Autodesk Inventor part; units mm, degrees
ref_plane "YZ Plane" through (0, 0, 0) normal (1, 0, 0) x (0, 1, 0)
ref_plane "XZ Plane" through (0, 0, 0) normal (0, 1, 0) x (-1, 0, 0)
ref_plane "XY Plane" through (0, 0, 0) normal (0, 0, 1) x (1, 0, 0)
sketch "Sketch1" plane through (0, 0, 0) normal (0, 0, 1) x (1, 0, 0)
  line L0 (-63.88, 42.74) -> (63.88, 42.74)
  line L1 (63.88, 42.74) -> (63.88, -42.74)
  line L2 (63.88, -42.74) -> (-63.88, -42.74)
  line L3 (-63.88, -42.74) -> (-63.88, 42.74)
  line L4 (63.88, 42.74) -> (-63.88, -42.74) construction
  point P0 (0, 0)
  point P1 (0, 0)
  dimension "d0" = 127.76
  dimension "d1" = 85.48
extrude "Extrusion1" add sketch "Sketch1" along normal blind 15
sketch "Sketch2" plane through (0, 0, 0) normal (0, 0, -1) x (-1, 0, 0)
  line L0 (-62.7, 41.65) -> (62.7, 41.65)
  line L1 (62.7, 41.65) -> (62.7, -41.65)
  line L2 (62.7, -41.65) -> (-62.7, -41.65)
  line L3 (-62.7, -41.65) -> (-62.7, 41.65)
  line L4 (62.7, 41.65) -> (-62.7, -41.65) construction
  point P0 (0, 0)
  point P1 (0, 0)
  dimension "d4" = 125.4
  dimension "d5" = 83.3
extrude "Extrusion2" cut sketch "Sketch2" against normal blind 2
sketch "Sketch3" plane through (0, 0, 2) normal (0, 0, -1) x (-1, 0, 0)
  line L0 (-55, 37.5) -> (55, 37.5)
  line L1 (55, 37.5) -> (55, -37.5)
  line L2 (55, -37.5) -> (-55, -37.5)
  line L3 (-55, -37.5) -> (-55, 37.5)
  line L4 (55, 37.5) -> (-55, -37.5) construction
  line L5 (-62.7, 41.65) -> (62.7, 41.65)
  line L6 (-62.7, -41.65) -> (-62.7, 41.65)
  line L7 (62.7, -41.65) -> (-62.7, -41.65)
  line L8 (62.7, 41.65) -> (62.7, -41.65)
  point P0 (0, 0)
  point P1 (0, 0)
  dimension "d8" = 75
  dimension "d9" = 110
extrude "Extrusion3" cut sketch "Sketch3" against normal blind 2
sketch "Sketch4" plane through (0, 0, 15) normal (0, 0, 1) x (1, 0, 0)
  line L0 (61.9, -40.8) -> (-61.9, -40.8)
  line L1 (-61.9, -40.8) -> (-61.9, 40.8)
  line L2 (-61.9, 40.8) -> (61.9, 40.8)
  line L3 (61.9, 40.8) -> (61.9, -40.8)
  line L4 (-61.9, -40.8) -> (61.9, 40.8) construction
  line L5 (63.88, 42.74) -> (-63.88, 42.74)
  line L6 (-63.88, 42.74) -> (-63.88, -42.74)
  line L7 (-63.88, -42.74) -> (63.88, -42.74)
  line L8 (63.88, -42.74) -> (63.88, 42.74)
  point P0 (0, 0)
  point P1 (0, 0)
  dimension "d12" = 123.8
  dimension "d13" = 81.6
extrude "Extrusion4" cut sketch "Sketch4" against normal blind 8.6
fillet "Fillet1" radius 3 8 edges at (62.7, 41.65, 2) (-62.7, 41.65, 2) (-62.7, -41.65, 2) (62.7, -41.65, 2) (63.88, -42.74, 3.2) (63.88, 42.74, 3.2) (-63.88, 42.74, 3.2) (-63.88, -42.74, 3.2)
fillet "Fillet2" radius 2 2 edges at (-61.9, -40.8, 10.7) (-61.9, 40.8, 10.7)
chamfer "Chamfer1" distance 6 angle 45 2 edges at (61.9, -40.8, 10.7) (61.9, 40.8, 10.7)
sketch "Sketch6" plane through (0, 0, 2) normal (0, 0, -1) x (-1, 0, 0)
  circle A0 centre (0, 0) radius 0.5
  dimension "d21" = 1
extrude "Extrusion5" add sketch "Sketch6" against normal blind 800
properties part number "well_plate"
Model file for the job. Use its own axes, mm. Coordinates: 2 decimals unless noted, no trailing zeros. Order: outer loops, then holes, each group sorted by start corner. A loop starts at its lowest first (then second) coordinate and runs counter-clockwise, first axis right, second up. Notation, with made-up numbers: (-22, 60.5) -> (32, 60.5) arc R14 ccw to (32, 77.5) -> close; hole circle Ø3 at (30.25, 67.25). An arc over 180 degrees is marked (long way). Return JSON: item names as keys, results as strings.
Item 1: Pin check, flat tips, straight feed: P1, Ø7, axis at x = 14.5, z = 12, coming from the -Y side; P2, Ø4, axis at x = -3, y = -7, coming from the -Z side; P3, Ø12, axis at y = 12, z = 603, coming from the +X side. Stop position of each tip, or through.
Model answer:
{"P1": "stops at y = -40.8", "P2": "stops at z = 2", "P3": "passes through"}
Item 2: Slice it at C-C (z = 395.5). Write the cut outline in (x, y).
Model answer:
{"outline": "circle Ø1 at (0, 0)"}
Item 3: Wall check: line 1 along Z through (x, y) = (-34, 30); line 2 along Z through (x, y) = (-47, -38). Give the ranges that are in metal, low to high. Write a range as from..to.
Model answer:
{"line 1": "z = 2..15", "line 2": "z = 4..15"}
Item 4: Slice it at B-B (x = -34.5). Write the cut outline in (y, z).
Model answer:
{"outline": "(-42.74, 0) -> (-41.65, 0) -> (-41.65, 4) -> (-37.5, 4) -> (-37.5, 2) -> (37.5, 2) -> (37.5, 4) -> (41.65, 4) -> (41.65, 0) -> (42.74, 0) -> (42.74, 6.4) -> (40.8, 6.4) -> (40.8, 15) -> (-40.8, 15) -> (-40.8, 6.4) -> (-42.74, 6.4) -> close"}
Item 5: Slice it at A-A (y = -8). Write the cut outline in (x, z).
Model answer:
{"outline": "(-63.88, 0) -> (-62.7, 0) -> (-62.7, 4) -> (-55, 4) -> (-55, 2) -> (55, 2) -> (55, 4) -> (62.7, 4) -> (62.7, 0) -> (63.88, 0) -> (63.88, 6.4) -> (61.9, 6.4) -> (61.9, 15) -> (-61.9, 15) -> (-61.9, 6.4) -> (-63.88, 6.4) -> close"}
Item 6: Mould opens along X. For faces 1 (the face through (0, 40, 4)), 2 (the face through (0, -41, 6.4)), 3 (the face through (1, 1, 2)) say: pulls with the +X half, pulls with the -X half, needs draft (parallel to the pull), parting line crosses it, or undercut.
Model answer:
{"face 1": "undercut", "face 2": "needs draft", "face 3": "undercut"}
